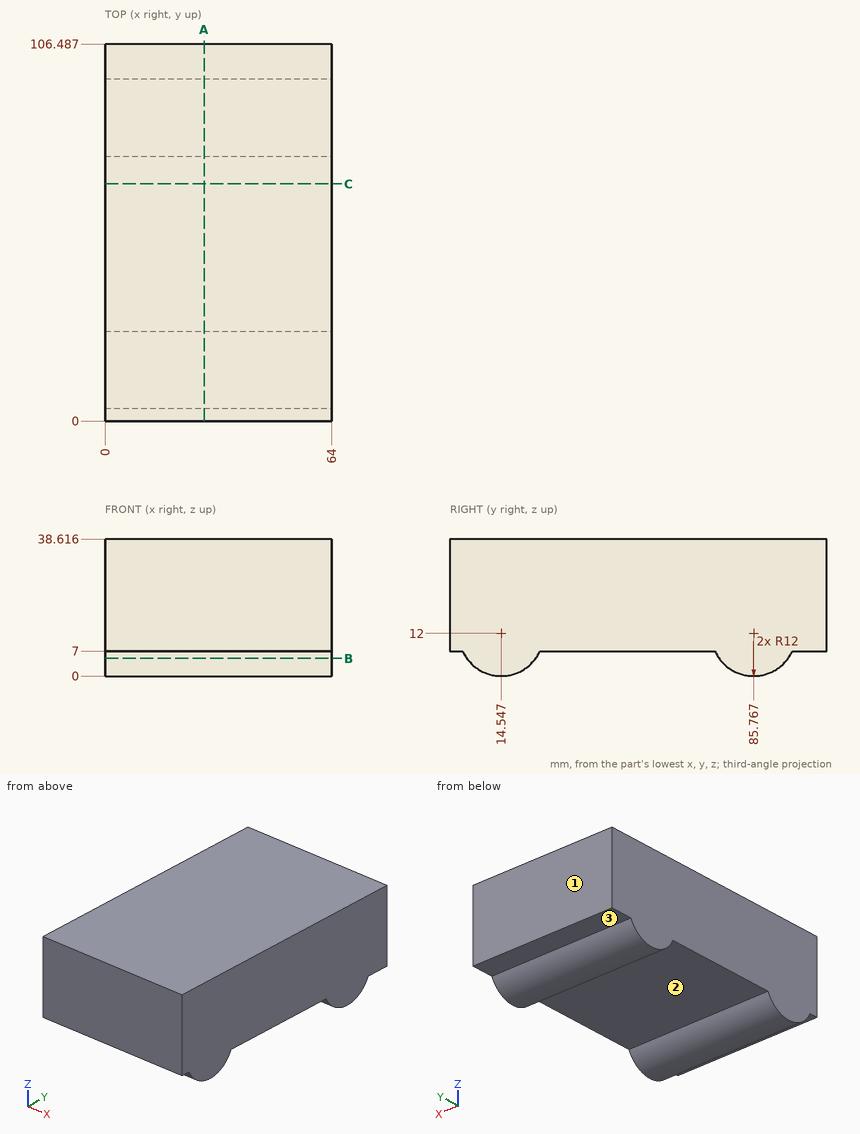
Answer from the drawing. Dimensions are ordinates in mm from the lowest x, y and z of the part. Round coordinates to 2 decimals unless told otherwise and drop trailing zeros. Write each loop counter-clockwise with the first axis right and the second up, starting at its lowest first coordinate (ties: lowest second). Pieces come first, ordered by that corner, then holes. Notation, with made-up numbers: (83.25, -23) -> (93.25, -23) arc R10 cw to (93.25, -11) -> close; hole circle Ø9 at (8, -26.75). An arc over 180 degrees is marked (long way). Answer in a Markdown table with one row per item. Add a question column.
1) Consider line 1 (Z direction, x = 17, y = 36.5); line 2 (Y direction, x = 60.5, z = 4) (1 decimal); line 3 (Z direction, x = 5, y = 86). Determine where each line is inside the solid, lowest interval first.
2) Find section B-B, the plane z = 5. Determine the outline of the cut face in (x, y) (1 decimal).
3) Find section C-C, the plane y = 67. Determine the outline of the cut face in (x, z).
4) Determine the mould class of the marked faces 1, 2 and 3 for opening direction Y: pulls with the +Y half, pulls with the -Y half, needs draft (parallel to the pull), parting line crosses it, or undercut.
5) Given P1, Ø1, axis at x = 10.5, y = 82, coming from the -Z side; P2, Ø1, axis at x = 7.5, y = 17.5, coming from the -Z side; P3, Ø1.1, axis at x = 28, y = 1, coming from the -Z side, each flat-ended and moving along its own axis, determine where each tip first touches the part or whether it passes through.
6) Find section A-A, the plane x = 28. Determine the outline of the cut face in (y, z).
Findings below:
| question | item | result |
|---|---|---|
| 1 | line 1 | 7 to 38.62 |
| 1 | line 2 | 5.6 to 23.5, 76.8 to 94.7 |
| 1 | line 3 | 0 to 38.62 |
| 2 | outline | (0, 4.8) -> (64, 4.8) -> (64, 24.3) -> (0, 24.3) -> close; (0, 76) -> (64, 76) -> (64, 95.5) -> (0, 95.5) -> close |
| 3 | outline | (0, 7) -> (64, 7) -> (64, 38.62) -> (0, 38.62) -> close |
| 4 | face 1 | pulls with the +Y half |
| 4 | face 2 | undercut |
| 4 | face 3 | needs draft |
| 5 | P1 | z = 0.45 |
| 5 | P2 | z = 0.25 |
| 5 | P3 | z = 7 |
| 6 | outline | (0, 7) -> (3.64, 7) arc R12 ccw to (25.46, 7) -> (74.86, 7) arc R12 ccw to (96.68, 7) -> (106.49, 7) -> (106.49, 38.62) -> (0, 38.62) -> close |
